Input: part model. Units: mm. Frame: model coordinates. A direction names the side the tool comes from. Coordinates: 2 decimals unless noted, no trailing zeros. Loops run counter-clockwise (first coordinate to the right, second up) from the corner with the lowest first, then second, coordinate; pieces in that order, holes last.
Item 1: Pull-direction query (X, two-part tool) for faces 3 (the cylindrical face through (138, 6, -123)), 4 (the flat face through (3, 23, -67)), 5 (the flat face through (137.83, 25.84, -131.2)), 6 (the cylindrical face through (8.867, 6.426, -63.319)); classes: released by +X, released by -X, zero draft, split by the parting line, or undercut.
Item 2: Section A-A on x = 217. Return loops of the section in (y, z), and give its area (3 significant figures).
Item 3: Reachability of faces 1 (the flat face through (269.055, 22.815, -65.52)), 2 (the flat face through (264.117, 27.745, -77.264)) from +Z, -Z, +X, -X, +Y, -Y: full face, straight path, thin tool, end or side. Return the list, or none.
Item 4: Contact query for flat-ended pins moving along their axis: P1, Ø12, axis at x = 229.5, z = -89.5, coming from the +Y side; P2, Ø3, axis at x = 121.5, y = 11, coming from the -Z side; P3, Ø5, axis at y = 18.5, z = -59, coming from the -X side. Output: stop coordinate, or through.
Item 5: Section B-B on y = 35.5. Return loops of the section in (x, z), and give its area (3 significant figures).
Item 6: Ray query, line 1 along Y through (x, z) = (257.5, -72.5); line 2 along X through (y, z) = (4, -63.5); line 3 along X through (y, z) = (20, -121.5). Return the intervals inside material, ascending.
```python
from build123d import *

# Parameters (mm, degrees)
SKETCH1_W           = 272
SKETCH1_H           = 134
BOSS_EXTRUDE2_DEPTH = 45
CUT_EXTRUDE8_DEPTH  = 300
CUT_EXTRUDE10_DEPTH = 300
CUT_EXTRUDE11_DEPTH = 40
CUT_EXTRUDE12_DEPTH = 5
CUT_EXTRUDE13_DEPTH = 5
FILLET1_R           = 10
FILLET2_R           = 5
FILLET3_R           = 10
FILLET5_R           = 2
FILLET6_R           = 2
FILLET7_R           = 2
BOSS_EXTRUDE3_DEPTH = 5
SKETCH18_W          = 22.005693375
SKETCH18_H          = 61.946637546
BOSS_EXTRUDE4_DEPTH = 5
SKETCH19_W          = 26.164660497
SKETCH19_H          = 10
BOSS_EXTRUDE5_DEPTH = 15
CUT_EXTRUDE15_DEPTH = 350
SKETCH22_W          = 22.005693375
SKETCH22_H          = 61.946637546
CUT_EXTRUDE16_DEPTH = 350
CUT_EXTRUDE17_DEPTH = 350
SKETCH26_W          = 366.999535542
SKETCH26_H          = 253.064882437
CUT_EXTRUDE18_DEPTH = 5
FILLET8_R           = 5
SKETCH27_W          = 167.245030015
SKETCH27_H          = 61.468608264
CUT_EXTRUDE19_DEPTH = 0.5
SKETCH28_W          = 245.78388014
SKETCH28_H          = 90.598055895
CUT_EXTRUDE20_DEPTH = 0.5
SKETCH29_W          = 367.28533999
SKETCH29_H          = 77.687990399
CUT_EXTRUDE21_DEPTH = 0.5


with BuildPart() as part:
    # Sketch1 → Boss-Extrude2 (new body)
    with BuildSketch(Plane(origin=(0, 0, 0), x_dir=(1, 0, 0), z_dir=(0, 1, 0))):
        with Locations((136, 67)):
            Rectangle(SKETCH1_W, SKETCH1_H)
    extrude(amount=BOSS_EXTRUDE2_DEPTH)

    # Sketch8 → Cut-Extrude8 (cut)
    with BuildSketch(Plane.ZY):
        Polygon((-134, 45), (-130, 45), (-134, 0), align=None)
    extrude(amount=-CUT_EXTRUDE8_DEPTH, mode=Mode.SUBTRACT)

    # Sketch9 → Cut-Extrude10 (cut)
    with BuildSketch(Plane.XZ):
        Polygon((0, -134), (5, -134), (0, 0), align=None)
        Polygon((272, -134), (267, -134), (272, 0), align=None)
    extrude(amount=-CUT_EXTRUDE10_DEPTH, mode=Mode.SUBTRACT)

    # Sketch11 → Cut-Extrude11 (cut)
    with BuildSketch(Plane(origin=(0, 45, 0), x_dir=(1, 0, 0), z_dir=(0, 1, 0))):
        Polygon((9.664179104, 125), (262.335820896, 125), (267, 0), (5, 0), align=None)
    extrude(amount=-CUT_EXTRUDE11_DEPTH, mode=Mode.SUBTRACT)

    # Sketch12 → Cut-Extrude12 (cut)
    with BuildSketch(Plane(origin=(0, 0, 0), x_dir=(-0.037287484326558824, 0, 0.9993045799517766), z_dir=(-0.9993045799517766, 0, -0.037287484326558824))):
        Polygon((0, 22.5), (-60.090467519, 45), (0, 45), align=None)
    extrude(amount=-CUT_EXTRUDE12_DEPTH, mode=Mode.SUBTRACT)

    # Sketch13 → Cut-Extrude13 (cut)
    with BuildSketch(Plane(origin=(271.621823035, 0, -10.135142651), x_dir=(-0.03728748432655886, 0, -0.9993045799517766), z_dir=(0.9993045799517766, 0, -0.03728748432655886))):
        Polygon((-10.142195737, 22.5), (49.948271782, 45), (-10.142195737, 45), align=None)
    extrude(amount=-CUT_EXTRUDE13_DEPTH, mode=Mode.SUBTRACT)

    # Fillet1
    fillet1_edges = [part.edges().sort_by_distance(p)[0] for p in [
        (2.5, 22.534904388, 0),
        (269.5, 22.534904388, 0),
    ]]
    fillet(fillet1_edges, radius=FILLET1_R)

    # Fillet2
    fillet2_edges = [part.edges().sort_by_distance(p)[0] for p in [
        (7.332089552, 5, -62.5),
        (136, 5, -125),
        (264.667910448, 5, -62.5),
    ]]
    fillet(fillet2_edges, radius=FILLET2_R)

    # Fillet3
    fillet3_edges = [part.edges().sort_by_distance(p)[0] for p in [
        (4.737146475, 45, -59.955525519),
        (267.262853525, 45, -59.955525519),
    ]]
    fillet(fillet3_edges, radius=FILLET3_R)

    # Fillet5
    fillet5_edges = [part.edges().sort_by_distance(p)[0] for p in [
        (136, 0, 0),
    ]]
    fillet(fillet5_edges, radius=FILLET5_R)

    # Fillet6
    fillet6_edges = [part.edges().sort_by_distance(p)[0] for p in [
        (136, 0, -134),
    ]]
    fillet(fillet6_edges, radius=FILLET6_R)

    # Fillet7
    fillet7_edges = [part.edges().sort_by_distance(p)[0] for p in [
        (136, 45, -130),
    ]]
    fillet(fillet7_edges, radius=FILLET7_R)

    # Sketch17 → Boss-Extrude3 (add)
    with BuildSketch(Plane.XZ):
        Polygon((0, 0), (242.409497269, 0), (294.229063893, 0), (294.229063893, -131.814336534), (242.409497269, -131.814336534), (0, -131.814336534), align=None)
    extrude(amount=BOSS_EXTRUDE3_DEPTH)

    # Sketch18 → Boss-Extrude4 (add)
    with BuildSketch(Plane(origin=(0, 0, 0), x_dir=(1, 0, 0), z_dir=(0, 1, 0))):
        with Locations((283.226217206, 100.841017761)):
            Rectangle(SKETCH18_W, SKETCH18_H)
    extrude(amount=BOSS_EXTRUDE4_DEPTH)

    # Sketch19 → Boss-Extrude5 (add)
    with BuildSketch(Plane(origin=(0, 0, -131.814336534), x_dir=(-1, 0, 0), z_dir=(0, 0, -1))):
        with Locations((-281.146733645, 0)):
            Rectangle(SKETCH19_W, SKETCH19_H)
    extrude(amount=BOSS_EXTRUDE5_DEPTH)

    # Sketch21 → Cut-Extrude15 (cut)
    with BuildSketch(Plane(origin=(294.229063893, 0, 0), x_dir=(0, 0, -1), z_dir=(1, 0, 0))):
        Polygon((69.867698988, -5), (131.814336534, 5), (146.814336534, 5), (146.814336534, -5), align=None)
    extrude(amount=-CUT_EXTRUDE15_DEPTH, mode=Mode.SUBTRACT)

    # Sketch22 → Cut-Extrude16 (cut)
    with BuildSketch(Plane(origin=(0, 5, 0), x_dir=(1, 0, 0), z_dir=(0, 1, 0))):
        with Locations((283.226217206, 100.841017761)):
            Rectangle(SKETCH22_W, SKETCH22_H)
    extrude(amount=-CUT_EXTRUDE16_DEPTH, mode=Mode.SUBTRACT)

    # Sketch24 → Cut-Extrude17 (cut)
    with BuildSketch(Plane(origin=(0, 0, 0), x_dir=(1, 0, 0), z_dir=(0, 1, 0))):
        Polygon((294.229063893, 69.867698988), (272.223370518, 69.867698988), (272.223370518, 100.841017761), (268.237275457, 100.841017761), (271.925373134, 2), (271.925373134, 0), (294.229063893, 0), align=None)
    extrude(amount=-CUT_EXTRUDE17_DEPTH, mode=Mode.SUBTRACT)

    # Sketch26 → Cut-Extrude18 (cut)
    with BuildSketch(Plane.XZ.offset(5)):
        with Locations((88.425605363, -126.532441219)):
            Rectangle(SKETCH26_W, SKETCH26_H)
    extrude(amount=-CUT_EXTRUDE18_DEPTH, mode=Mode.SUBTRACT)

    # Fillet8
    # the kernel refuses this fillet: 5 mm, written as the material it takes off along each edge
    with BuildSketch(Plane(origin=(276.867640222, 5, -133.555555556), x_dir=(0, 0.996072640692687, 0.08853979028378928), z_dir=(-1, 0, 0))) as fillet8_piece_1:
        with BuildLine():
            CenterArc((3.94042259, -5), FILLET8_R, 90, 49.222455221)
            Line((0.154167167, -1.734380629), (0.078442059, -1.669068242))
            ThreePointArc((0.078442059, -1.669068242), (-0.022523681, -0.876044294), (-0.099607264, -0.008853979))
            Line((-0.099607264, -0.008853979), (0, 0.1))
            Line((0, 0.1), (3.94042259, 0.1))
            Line((3.94042259, 0.1), (3.94042259, 0))
        make_face()
    extrude(amount=281.735280444, mode=Mode.SUBTRACT)

    # Sketch27 → Cut-Extrude19 (cut)
    with BuildSketch(Plane(origin=(271.621823035, 0, -10.135142651), x_dir=(-0.03728748432655886, 0, -0.9993045799517766), z_dir=(0.9993045799517766, 0, -0.03728748432655886))):
        with Locations((55.876182623, 22.646622557)):
            Rectangle(SKETCH27_W, SKETCH27_H)
    extrude(amount=-CUT_EXTRUDE19_DEPTH, mode=Mode.SUBTRACT)

    # Sketch28 → Cut-Extrude20 (cut)
    with BuildSketch(Plane(origin=(0, 0, 0), x_dir=(-0.037287484326558824, 0, 0.9993045799517766), z_dir=(-0.9993045799517766, 0, -0.037287484326558824))):
        with Locations((-84.953882452, 20.133440951)):
            Rectangle(SKETCH28_W, SKETCH28_H)
    extrude(amount=-CUT_EXTRUDE20_DEPTH, mode=Mode.SUBTRACT)

    # Sketch29 → Cut-Extrude21 (cut)
    with BuildSketch(Plane(origin=(0, 11.817736404, -132.949534542), x_dir=(-1, 0, 0), z_dir=(0, 0.08853979028379444, -0.9960726406926865))):
        with Locations((-152.32774441, 16.969098034)):
            Rectangle(SKETCH29_W, SKETCH29_H)
    extrude(amount=-CUT_EXTRUDE21_DEPTH, mode=Mode.SUBTRACT)


solid = part.part
```
Results found:
1. face 3: undercut
1. face 4: released by -X
1. face 5: zero draft
1. face 6: undercut
2. outline: (0, -100.84) - (5, -131.81) arc R5 ccw to (6.71, -132.9) - (44.45, -129.55) arc R2 ccw to (45, -128.17) - (45, -125) - (10, -125) arc R5 cw to (5, -120) - (5, 0) - (2, 0) arc R2 ccw to (0, -2) - close
2. area: 836 mm2
3. face 1: -Z, +X, +Y, -Y
3. face 2: +Z, +Y
4. P1: stops at y = 5
4. P2: stops at z = -132.65
4. P3: stops at x = 2.61
5. outline: (1.79, -34.68) - (5.36, -130.34) - (266.64, -130.34) - (270.21, -34.68) - (265.71, -34.51) - (262.34, -125) - (9.66, -125) - (6.29, -34.51) - close
5. area: 2,210 mm2
6. line 1: y = 0 to 5
6. line 2: x = 2.87 to 269.13
6. line 3: x = 5.03 to 9.53, 262.47 to 266.97
